from build123d import *

# Parameters (mm, degrees)
F1_DEPTH = 63.5
F0_W     = 25.4
F0_H     = 19.05
F2_DEPTH = 25.4
F3_DEPTH = 7.9375
F5_R     = 6.35


with BuildPart() as f1:
    # F0 (on Front) → F1 (new body, symmetric)
    with BuildSketch(Plane.XZ):
        Polygon((-41.275, 9.525), (-41.275, -9.525), (41.275, -9.525), (41.275, 9.525), (22.225, 9.525), align=None)
    extrude(amount=F1_DEPTH, both=True)

    # F0 (on Front) → F2 (join, symmetric)
    with BuildSketch(Plane.XZ):
        with Locations((73.025, 52.4002)):
            Rectangle(F0_W, F0_H)
        with BuildLine():
            Line((22.225, 9.525), (41.275, 9.525))
            Line((41.275, 9.525), (41.275, 27.0002))
            ThreePointArc((41.275, 27.0002), (45.9246798487, 38.2255201513), (57.15, 42.8752))
            Line((57.15, 42.8752), (60.325, 42.8752))
            Line((60.325, 42.8752), (60.325, 61.9252))
            Line((60.325, 61.9252), (57.15, 61.9252))
            add(Edge.make_bspline(
                [(56.4515488483, 61.9182152785), (56.6842963027, 61.9210832952), (56.9171147806, 61.9234123626), (57.15, 61.9252)],
                knots=[110.9913484912, 110.9913484912, 110.9913484912, 110.9913484912, 111.5045361635, 111.5045361635, 111.5045361635, 111.5045361635], degree=3))
            ThreePointArc((56.4515488483, 61.9182152785), (32.2085783136, 51.4477174458), (22.225, 27.0002))
            Line((22.225, 27.0002), (22.225, 9.525))
        make_face()
    extrude(amount=F2_DEPTH, both=True)

    # F0 (on Front) → F3 (join, symmetric)
    with BuildSketch(Plane.XZ):
        with BuildLine():
            add(Edge.make_bspline(
                [(-41.275, 9.525), (-40.9026709166, 35.4675879968), (6.1133291004, 61.2979255596), (56.4515488483, 61.9182152785)],
                knots=[0, 0, 0, 0, 110.9913484912, 110.9913484912, 110.9913484912, 110.9913484912], degree=3))
            Line((-41.275, 9.525), (22.225, 9.525))
            Line((22.225, 9.525), (22.225, 27.0002))
            ThreePointArc((22.225, 27.0002), (32.2085783136, 51.4477174458), (56.4515488483, 61.9182152785))
        make_face()
    extrude(amount=F3_DEPTH, both=True)

    # F0 (on Front) → F4 (revolve)
    with BuildSketch(Plane.XZ):
        Polygon((85.725, 66.675), (85.725, 61.9252), (85.725, 42.8752), (85.725, 38.1), (111.125, 38.1), (111.125, 66.675), align=None)
    revolve(axis=Axis((85.725, 0, 52.3875), (0, 0, 1)))

    # F5
    f5_edges = [f1.edges().sort_by_distance(p)[0] for p in [
        (41.275, -63.5, 0),
        (-41.275, -63.5, 0),
        (41.275, 63.5, 0),
        (-41.275, 63.5, 0),
    ]]
    fillet(f5_edges, radius=F5_R)


solid = f1.part
Verification items for the finished model (mm, model axes). A direction names the side the tool comes from. Coordinates: 2 decimals unless noted, no trailing zeros. Write each loop counter-clockwise with the first axis right and the second up, starting at its lowest first coordinate (ties: lowest second). Pieces come first, ordered by that corner, then holes. Notation, with made-up numbers: (-33, 77) - (6, 77) arc R30 ccw to (6, 102) - close; hole circle Ø1 at (87.5, 71). An arc over 180 degrees is marked (long way). Answer as a JSON object with one key per item and string values.
(1) Tool access check on faces 4 (the flat face through (60, -2, 61.925)), 5 (the flat face through (41.275, -1, 4)), 6 (the flat face through (46, 25.4, 42)), 7 (the flat face through (46, -25.4, 42)). Record the directions out of +Z, -Z, +X, -X, +Y, -Y that give a thin tool (end or side, any length) a straight path to the whole face; none if there is none.
Report:
{"face 4": "+Z, -X", "face 5": "-Z, +X, +Y, -Y", "face 6": "+Z, +X, -X, +Y", "face 7": "+Z, +X, -X, -Y"}
(2) Cross-section at B-B on x = 82. Record the cut outline in (y, z) (3 decimals).
Report:
{"outline": "(-25.4, 42.875) - (-25.125, 42.875) - (-25.125, 38.1) - (25.125, 38.1) - (25.125, 42.875) - (25.4, 42.875) - (25.4, 61.925) - (25.125, 61.925) - (25.125, 66.675) - (-25.125, 66.675) - (-25.125, 61.925) - (-25.4, 61.925) - close"}
(3) Thickness scan on line 1 along Z through (x, y) = (-5, -11) (3 decimals); line 2 along X through (y, z) = (22, 26) (3 decimals); line 3 along X through (y, z) = (-5, 0) (3 decimals). Record the ranges inside material, lowest first.
Report:
{"line 1": "-9.525 to 9.525", "line 2": "22.225 to 41.275", "line 3": "-41.275 to 41.275"}
(4) Mould release check, pull along X, two halves, no side actions. Record for faces 1 (the flat face through (86, 0, 38.1)), 2 (the flat face through (60, 2, 42.875)), 3 (the cylindrical face through (32.48, 16.55, 51.72)): pulls with the +X half, pulls with the -X half, needs draft (parallel to the pull), parting line crosses it, or undercut.
Report:
{"face 1": "needs draft", "face 2": "undercut", "face 3": "pulls with the -X half"}
(5) Gauge pin test, flat ends, axial feed: pin 1 Ø15.5 at (x, z) = (-15.5, 41) entering from +Y; pin 2 Ø2 at (x, y) = (-3, 37.5) entering from +Z (3 decimals); pin 3 Ø4 at (y, z) = (-7, 40.5) entering from +X. Record the tip position at first contact, or that the pin passes through.
Report:
{"pin 1": "y = 7.94", "pin 2": "z = 9.525", "pin 3": "x = 110.63"}
(6) Cross-section at C-C on y = 36. Record the cut outline in (x, z) (3 decimals), plus the area to 3 significant figures.
Report:
{"outline": "(-41.275, -9.525) - (41.275, -9.525) - (41.275, 9.525) - (-41.275, 9.525) - close", "area": "1,570 mm^2"}
(7) Cross-section at A-A on z = 4.5. Record the cut outline in (x, y) (3 decimals), plus the area to 3 significant figures.
Report:
{"outline": "(-41.275, -57.15) arc R6.35 ccw to (-34.925, -63.5) - (34.925, -63.5) arc R6.35 ccw to (41.275, -57.15) - (41.275, 57.15) arc R6.35 ccw to (34.925, 63.5) - (-34.925, 63.5) arc R6.35 ccw to (-41.275, 57.15) - close", "area": "10,400 mm^2"}
